Source: CAD feature listing. Evaluate the final solid. Frame: model axes, mm. Face numbers are marked on the shaded views. Round coordinates to 2 decimals unless told otherwise and drop trailing zeros. Write each loop counter-clockwise with the first axis right and the second up, starting at its lowest first coordinate (ties: lowest second). Pieces come first, ordered by that corner, then holes. Notation, with made-up numbers: M -33,24 L 11,24 A32 ccw 11,58 Z; hole C 26,38 d7. An arc over 180 degrees is marked long. Answer in a Markdown table with one row per item.
from build123d import *

# Parameters (mm, degrees)
BOSS_EXTRUDE1_DEPTH = 5
SKETCH2_W           = 4
SKETCH2_H           = 9
SKETCH2_W_2         = 9
SKETCH2_H_2         = 4
BOSS_EXTRUDE2_DEPTH = 15
SKETCH3_W           = 5
SKETCH3_H           = 25.4
SKETCH3_W_2         = 25.4
SKETCH3_H_2         = 5
BOSS_EXTRUDE3_DEPTH = 5
CUT_EXTRUDE1_DEPTH  = 173.699160392
CUT_EXTRUDE2_DEPTH  = 173.699160392
FILLET1_R           = 1
FILLET2_R           = 1.5
SKETCH6_R           = 1.55
CUT_EXTRUDE3_DEPTH  = 5
SKETCH7_R           = 1.55
CUT_EXTRUDE4_DEPTH  = 5
FILLET3_R           = 1.5
FILLET4_R           = 1.5


with BuildPart() as part:
    # Sketch1 → Boss-Extrude1 (new body)
    with BuildSketch(Plane(origin=(0, 0, 0), x_dir=(1, 0, 0), z_dir=(0, 1, 0))):
        with BuildLine():
            Line((5, 0), (135, 0))
            ThreePointArc((135, 0), (138.535533906, 1.464466094), (140, 5))
            Line((140, 5), (140, 95))
            ThreePointArc((140, 95), (138.535533906, 98.535533906), (135, 100))
            Line((135, 100), (5, 100))
            ThreePointArc((5, 100), (1.464466094, 98.535533906), (0, 95))
            Line((0, 95), (0, 5))
            ThreePointArc((0, 5), (1.464466094, 1.464466094), (5, 0))
        make_face()
    extrude(amount=BOSS_EXTRUDE1_DEPTH)

    # Sketch2 → Boss-Extrude2 (add)
    with BuildSketch(Plane.XZ):
        with Locations((14, -46.5)):
            Rectangle(SKETCH2_W, SKETCH2_H)
        with Locations((123.5, -57)):
            Rectangle(SKETCH2_W_2, SKETCH2_H_2)
    extrude(amount=BOSS_EXTRUDE2_DEPTH)

    # Sketch3 → Boss-Extrude3 (add)
    with BuildSketch(Plane(origin=(0, 5, 0), x_dir=(1, 0, 0), z_dir=(0, 1, 0))):
        with Locations((2.5, 75)):
            Rectangle(SKETCH3_W, SKETCH3_H)
        with Locations((2.5, 25)):
            Rectangle(SKETCH3_W, SKETCH3_H)
        with Locations((137.5, 75)):
            Rectangle(SKETCH3_W, SKETCH3_H)
        with Locations((137.5, 25)):
            Rectangle(SKETCH3_W, SKETCH3_H)
        with Locations((35, 97.5)):
            Rectangle(SKETCH3_W_2, SKETCH3_H_2)
        with Locations((105, 97.5)):
            Rectangle(SKETCH3_W_2, SKETCH3_H_2)
        with Locations((35, 2.5)):
            Rectangle(SKETCH3_W_2, SKETCH3_H_2)
        with Locations((105, 2.5)):
            Rectangle(SKETCH3_W_2, SKETCH3_H_2)
    extrude(amount=BOSS_EXTRUDE3_DEPTH)

    # Sketch4 → Cut-Extrude1 (cut, through all)
    with BuildSketch(Plane.ZY):
        with BuildLine():
            Line((-84.5, 8.5), (-65.5, 8.5))
            ThreePointArc((-65.5, 8.5), (-65.146446609, 8.353553391), (-65, 8))
            Line((-65, 8), (-65, 7))
            ThreePointArc((-65, 7), (-65.146446609, 6.646446609), (-65.5, 6.5))
            Line((-65.5, 6.5), (-84.5, 6.5))
            ThreePointArc((-84.5, 6.5), (-84.853553391, 6.646446609), (-85, 7))
            Line((-85, 7), (-85, 8))
            ThreePointArc((-85, 8), (-84.853553391, 8.353553391), (-84.5, 8.5))
        make_face()
        with BuildLine():
            Line((-34.5, 8.5), (-15.5, 8.5))
            ThreePointArc((-15.5, 8.5), (-15.146446609, 8.353553391), (-15, 8))
            Line((-15, 8), (-15, 7))
            ThreePointArc((-15, 7), (-15.146446609, 6.646446609), (-15.5, 6.5))
            Line((-15.5, 6.5), (-34.5, 6.5))
            ThreePointArc((-34.5, 6.5), (-34.853553391, 6.646446609), (-35, 7))
            Line((-35, 7), (-35, 8))
            ThreePointArc((-35, 8), (-34.853553391, 8.353553391), (-34.5, 8.5))
        make_face()
    extrude(amount=-CUT_EXTRUDE1_DEPTH, mode=Mode.SUBTRACT)

    # Sketch8 → Cut-Extrude2 (cut, through all)
    with BuildSketch(Plane.XY):
        with BuildLine():
            Line((25.5, 8.5), (44.5, 8.5))
            ThreePointArc((44.5, 8.5), (44.853553391, 8.353553391), (45, 8))
            Line((45, 8), (45, 7))
            ThreePointArc((45, 7), (44.853553391, 6.646446609), (44.5, 6.5))
            Line((44.5, 6.5), (25.5, 6.5))
            ThreePointArc((25.5, 6.5), (25.146446609, 6.646446609), (25, 7))
            Line((25, 7), (25, 8))
            ThreePointArc((25, 8), (25.146446609, 8.353553391), (25.5, 8.5))
        make_face()
        with BuildLine():
            Line((95.5, 8.5), (114.5, 8.5))
            ThreePointArc((114.5, 8.5), (114.853553391, 8.353553391), (115, 8))
            Line((115, 8), (115, 7))
            ThreePointArc((115, 7), (114.853553391, 6.646446609), (114.5, 6.5))
            Line((114.5, 6.5), (95.5, 6.5))
            ThreePointArc((95.5, 6.5), (95.146446609, 6.646446609), (95, 7))
            Line((95, 7), (95, 8))
            ThreePointArc((95, 8), (95.146446609, 8.353553391), (95.5, 8.5))
        make_face()
    extrude(amount=-CUT_EXTRUDE2_DEPTH, mode=Mode.SUBTRACT)

    # Fillet1
    fillet1_edges = [part.edges().sort_by_distance(p)[0] for p in [
        (92.3, 10, -97.5),
        (117.7, 10, -97.5),
        (22.3, 10, -2.5),
        (47.7, 10, -2.5),
        (92.3, 10, -2.5),
        (117.7, 10, -2.5),
        (2.5, 10, -62.3),
        (2.5, 10, -87.7),
        (137.5, 10, -87.7),
        (137.5, 10, -62.3),
        (2.5, 10, -12.3),
        (2.5, 10, -37.7),
        (137.5, 10, -37.7),
        (137.5, 10, -12.3),
        (22.3, 10, -97.5),
        (47.7, 10, -97.5),
    ]]
    fillet(fillet1_edges, radius=FILLET1_R)

    # Fillet2
    fillet2_edges = [part.edges().sort_by_distance(p)[0] for p in [
        (92.3, 5, -97.5),
        (117.7, 5, -97.5),
        (22.3, 5, -2.5),
        (47.7, 5, -2.5),
        (92.3, 5, -2.5),
        (117.7, 5, -2.5),
        (2.5, 5, -62.3),
        (2.5, 5, -87.7),
        (137.5, 5, -87.7),
        (137.5, 5, -62.3),
        (2.5, 5, -12.3),
        (2.5, 5, -37.7),
        (137.5, 5, -37.7),
        (137.5, 5, -12.3),
        (22.3, 5, -97.5),
        (47.7, 5, -97.5),
    ]]
    fillet(fillet2_edges, radius=FILLET2_R)

    # Sketch6 → Cut-Extrude3 (cut)
    with BuildSketch(Plane.ZY.offset(-12)):
        with Locations((-46.5, -11)):
            Circle(SKETCH6_R)
    extrude(amount=-CUT_EXTRUDE3_DEPTH, mode=Mode.SUBTRACT)

    # Sketch7 → Cut-Extrude4 (cut)
    with BuildSketch(Plane.XY.offset(-55)):
        with Locations((123.5, -11)):
            Circle(SKETCH7_R)
    extrude(amount=-CUT_EXTRUDE4_DEPTH, mode=Mode.SUBTRACT)

    # Fillet3
    fillet3_edges = [part.edges().sort_by_distance(p)[0] for p in [
        (14, -15, -51),
        (14, -15, -42),
        (119, -15, -57),
        (128, -15, -57),
    ]]
    fillet(fillet3_edges, radius=FILLET3_R)

    # Fillet4
    fillet4_edges = [part.edges().sort_by_distance(p)[0] for p in [
        (14, 0, -51),
        (14, 0, -42),
        (119, 0, -57),
        (128, 0, -57),
    ]]
    fillet(fillet4_edges, radius=FILLET4_R)


solid = part.part
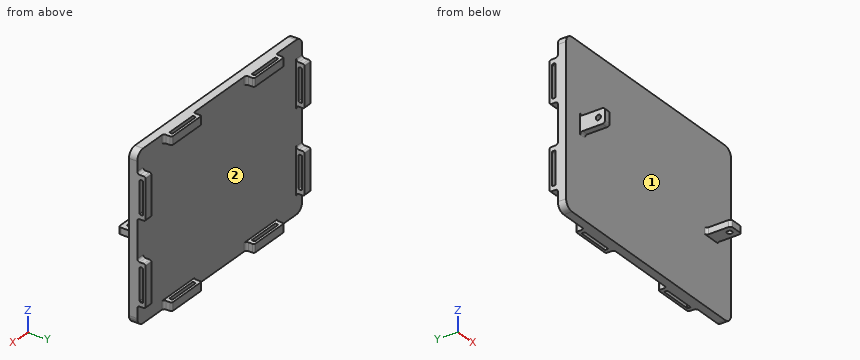
Q1. Section A-A (z = -46.5). Return loops of the section in (x, y), and give its area (3 significant figures).
Solutions:
| item | result |
|---|---|
| outline | M 0,0 L 12,0 L 12,-9.45 L 16,-9.45 L 16,0 L 140,0 L 140,5 L 0,5 Z; M 12,-15 L 16,-15 L 16,-12.55 L 12,-12.55 Z |
| area | 748 mm2 |
Q2. Section D-D (z = -75). Return loops of the section in (x, y), and give its area (3 significant figures).
Solutions:
| item | result |
|---|---|
| outline | M 0,0 L 140,0 L 140,6.5 L 135,6.5 L 135,5 L 5,5 L 5,6.5 L 0,6.5 Z; M 0,8.5 L 5,8.5 L 5,10 L 0,10 Z; M 135,8.5 L 140,8.5 L 140,10 L 135,10 Z |
| area | 730 mm2 |
Q3. Section B-B (x = 123.5). Return loops of the section in (y, z).
Solutions:
| item | result |
|---|---|
| outline | M -15,-59 L -12.55,-59 L -12.55,-55 L -15,-55 Z; M -9.45,-59 L 0,-59 L 0,-100 L 5,-100 L 5,0 L 0,0 L 0,-55 L -9.45,-55 Z |
Q4. Material intervals for probe 1 along Y at (x, z) = (123.5, -57.55); probe 2 along Y at (x, z) = (60.5, -63.5); probe 3 along X at (y, z) = (9, -31), sorted ascending.
Solutions:
| item | result |
|---|---|
| probe 1 | y = -15 to -12.55, -9.45 to 5 |
| probe 2 | y = 0 to 5 |
| probe 3 | x = 0 to 5, 135 to 140 |
Q5. Contact query for flat-ended pins moving along their axis: pin 1 Ø2 at (y, z) = (-6.5, -58) entering from -X; pin 2 Ø9.5 at (y, z) = (-7.5, -45.5) entering from -X; pin 3 Ø0.8 at (y, z) = (8.5, -2.5) entering from -X. Output: stop coordinate, or through.
Solutions:
| item | result |
|---|---|
| pin 1 | stops at x = 119 |
| pin 2 | stops at x = 12 |
| pin 3 | stops at x = 22.3 |
Q6. Pull-direction query (X, two-part tool) for the marked faces 1 and 2; classes: pulls with the +X half, pulls with the -X half, needs draft (parallel to the pull), parting line crosses it, or undercut.
Solutions:
| item | result |
|---|---|
| face 1 | needs draft |
| face 2 | undercut |
Q7. Section C-C (y = -11). Return loops of the section in (x, z), and give its area (3 significant figures).
Solutions:
| item | result |
|---|---|
| outline | M 12,-51 L 16,-51 L 16,-48.05 L 12,-48.05 Z; M 12,-44.95 L 16,-44.95 L 16,-42 L 12,-42 Z; M 119,-59 L 121.95,-59 L 121.95,-55 L 119,-55 Z; M 125.05,-59 L 128,-59 L 128,-55 L 125.05,-55 Z |
| area | 47.2 mm2 |
